from build123d import *

# Parameters (mm, degrees)
F1_DEPTH = 12.7
F2_W     = 2.54
F2_H     = 12.7
F3_DEPTH = 12.7
F4_R     = 1.27
F5_DEPTH = 25.4
F6_R     = 1.27
F7_DEPTH = 25.4
F8_R     = 5.08


with BuildPart() as f1:
    # F0 (on Top) → F1 (new body)
    with BuildSketch(Plane.XY):
        Polygon((-38.1, -21.997045), (38.1, -21.997045), (0, 43.994091), align=None)
    extrude(amount=F1_DEPTH)

    # F2 (on face) → F3 (join)
    with BuildSketch(Plane.XZ.offset(21.997045)):
        with Locations((-16.51, 6.35)):
            Rectangle(F2_W, F2_H)
        with Locations((16.51, 6.35)):
            Rectangle(F2_W, F2_H)
    extrude(amount=F3_DEPTH)

    # F4 (on face) → F5 (cut)
    with BuildSketch(Plane.YZ.offset(17.78)):
        with Locations((-28.347045, 6.35)):
            Circle(F4_R)
    extrude(amount=-F5_DEPTH, mode=Mode.SUBTRACT)

    # F6 (on face) → F7 (cut)
    with BuildSketch(Plane(origin=(-17.78, 0, 0), x_dir=(0, -1, 0), z_dir=(-1, 0, 0))):
        with Locations((28.347045, 6.35)):
            Circle(F6_R)
    extrude(amount=-F7_DEPTH, mode=Mode.SUBTRACT)

    # F8
    f8_edges = [f1.edges().sort_by_distance(p)[0] for p in [
        (-16.51, -34.697045, 12.7),
        (-16.51, -34.697045, 0),
        (16.51, -34.697045, 0),
        (16.51, -34.697045, 12.7),
    ]]
    fillet(f8_edges, radius=F8_R)


solid = f1.part
Design review of the part built by this model. Coordinates are the model's own, in mm. A direction names the side the tool comes from. Coordinates: 2 decimals unless noted, no trailing zeros. Order: outer loops, then holes, each group sorted by start corner. A loop starts at its lowest first (then second) coordinate and runs counter-clockwise, first axis right, second up. Notation, with made-up numbers: (-10.5, 70) -> (29.5, 70) arc R25 ccw to (29.5, 107) -> close; hole circle Ø5 at (2.5, 14). An arc over 180 degrees is marked (long way). One line per item, written item: value.
1) We need section C-C, the plane z = 1. Give the boundary of the cut face in (x, y).
Output values:
outline: (-38.1, -22) -> (-17.78, -22) -> (-17.78, -32.64) -> (-15.24, -32.64) -> (-15.24, -22) -> (15.24, -22) -> (15.24, -32.64) -> (17.78, -32.64) -> (17.78, -22) -> (38.1, -22) -> (0, 43.99) -> close
2) We need section D-D, the plane x = -32. Give the boundary of the cut face in (y, z), then the cut area to 3 significant figures.
Output values:
outline: (-22, 0) -> (-11.43, 0) -> (-11.43, 12.7) -> (-22, 12.7) -> close
area: 134 mm2
3) Draft analysis for pull direction Z (two halves, no side actions). For faces 6 (the face through (-15.24, -26.8, 6.3)), 7 (the face through (-16.53, -28.18, 7.61)), 8 (the face through (-16.49, -33.17, 1.45)), state which applies: +Z half, -Z half, draft (parallel to the pull), parting line (faces both ways), or undercut.
Output values:
face 6: draft
face 7: undercut
face 8: -Z half
4) Clearance check with flat-ended pins moving along their axes: P1, Ø6.5, axis at x = 1, z = 4, coming from the -Y side; P2, Ø6.5, axis at y = -30, z = 4.5, coming from the -X side; P3, Ø6.5, axis at y = -30.5, z = 6.5, coming from the +X side; P4, Ø1.5, axis at y = -28.35, z = 6.35, coming from the -X side. State where each tip first meets the part, or that it passes through.
Output values:
P1: stops at y = -22
P2: stops at x = -17.78
P3: stops at x = 17.78
P4: passes through
5) We need section A-A, the plane z = 6.35. Give the boundary of the cut face in (x, y).
Output values:
outline: (-38.1, -22) -> (-17.78, -22) -> (-17.78, -27.08) -> (-15.24, -27.08) -> (-15.24, -22) -> (15.24, -22) -> (15.24, -27.08) -> (17.78, -27.08) -> (17.78, -22) -> (38.1, -22) -> (0, 43.99) -> close; (-17.78, -34.7) -> (-15.24, -34.7) -> (-15.24, -29.62) -> (-17.78, -29.62) -> close; (15.24, -34.7) -> (17.78, -34.7) -> (17.78, -29.62) -> (15.24, -29.62) -> close
6) We need section B-B, the plane y = -28.5. Give the boundary of the cut face in (x, z).
Output values:
outline: (-17.78, 0) -> (-15.24, 0) -> (-15.24, 5.09) -> (-17.78, 5.09) -> close; (-17.78, 7.61) -> (-15.24, 7.61) -> (-15.24, 12.7) -> (-17.78, 12.7) -> close; (15.24, 0) -> (17.78, 0) -> (17.78, 5.09) -> (15.24, 5.09) -> close; (15.24, 7.61) -> (17.78, 7.61) -> (17.78, 12.7) -> (15.24, 12.7) -> close
7) Machinability: for faces 1 (the face through (17.78, -26.8, 6.3)), 2 (the face through (15.24, -26.8, 6.3)), 3 (the face through (-28, -21.997, 6)), 4 (the face through (-18.783, 11.46, 6.261)), 5 (the face through (16.53, -33.17, 1.45)), which of the approach directions +Z, -Z, +X, -X, +Y, -Y give a long, thin tool a straight path to every point of the face, cutting with its end or side? Answer none if there is none.
Output values:
face 1: +Z, -Z, +X, -Y
face 2: +Z, -Z, -Y
face 3: +Z, -Z, -X, -Y
face 4: +Z, -Z, -X, +Y
face 5: -Z, +X, -X, -Y
8) To check wall thickness, follow probe 1 along X at (y, z) = (-30, 9); probe 2 along Y at (x, z) = (-19, 2.75); probe 3 along X at (y, z) = (13, 4.5). State the ranges of each line that lie inside material, in increasing order. Write a range as [from, to].
Output values:
probe 1: x = [-17.78, -15.24], [15.24, 17.78]
probe 2: y = [-22, 11.09]
probe 3: x = [-17.89, 17.89]
